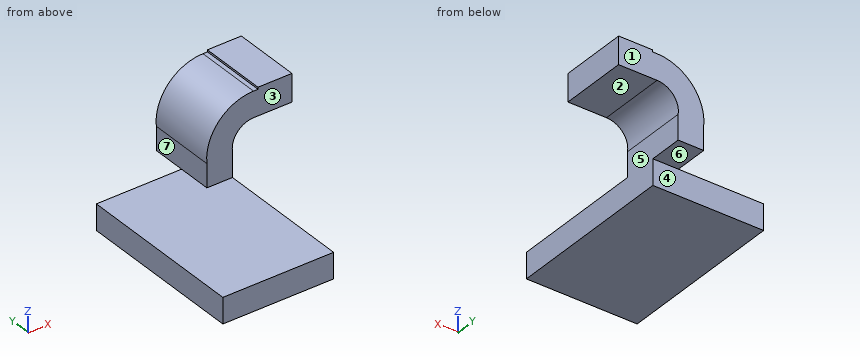
from build123d import *

# Parameters (mm, degrees)
F1_DEPTH = 127
F2_DEPTH = 25.4


with BuildPart() as f1:
    # F0 (on Front) → F1 (new body)
    with BuildSketch(Plane.XZ):
        Polygon((41.275, -9.525), (41.275, 9.525), (22.225, 9.525), (-41.275, 9.525), (-41.275, -9.525), align=None)
    extrude(amount=F1_DEPTH)

    # F0 (on Front) → F2 (join, symmetric)
    with BuildSketch(Plane.XZ):
        with BuildLine():
            Line((22.225, 9.525), (41.275, 9.525))
            Line((41.275, 9.525), (41.275, 27.979645))
            ThreePointArc((41.275, 27.979645), (44.97222, 40.659064), (56.982722, 46.153145))
            Line((56.982722, 46.153145), (60.325, 46.153145))
            Line((60.325, 46.153145), (60.325, 65.203145))
            Line((60.325, 65.203145), (56.982722, 65.203145))
            ThreePointArc((56.982722, 65.203145), (31.108074, 53.735729), (22.225, 26.863997))
            Line((22.225, 26.863997), (22.225, 9.525))
        make_face()
        Polygon((60.325, 65.203145), (60.325, 46.153145), (85.689964, 46.153145), (85.600682, 66.675), (60.325, 66.675), align=None)
    extrude(amount=F2_DEPTH, both=True)


solid = f1.part
The model under review builds one solid part; all positions refer to its coordinate system, in mm. Face numbers are marked on the shaded views. A direction names the side the tool comes from. Round coordinates to 2 decimals unless told otherwise and drop trailing zeros. Loops run counter-clockwise (first coordinate to the right, second up) from the corner with the lowest first, then second, coordinate; pieces in that order, holes last. Notation, with made-up numbers: (80.25, 15.5) -> (84.25, 15.5) arc R16 cw to (84.25, 32.5) -> close; hole circle Ø5 at (14, -11). An arc over 180 degrees is marked (long way). One line per question, with ' | ' between items. Start each with the question number.
Item 1: Add section C-C, the plane z = 18. Write out the cut boundary in (x, y) (3 decimals).
Item 2: Draft analysis for pull direction Z (two halves, no side actions). For the marked faces 5, 6 and 7, state which applies: +Z half, -Z half, draft (parallel to the pull), parting line (faces both ways), or undercut.
Item 3: Machinability: for the marked faces 1, 2, 3 and 4, which of the approach directions +Z, -Z, +X, -X, +Y, -Y give a long, thin tool a straight path to every point of the face, cutting with its end or side? Answer none if there is none.
Item 4: Wall thickness on line 1 along Z through (x, y) = (37.5, -52) (3 decimals); line 2 along X through (y, z) = (-118, 9) (3 decimals); line 3 along Y through (x, z) = (23.5, -5.5): over which ranges is each line inside the solid? List them lowest first. Write a range as [from, to].
Item 5: Add section B-B, the plane x = -27.5. Write out the cut boundary in (y, z) (3 decimals), then the cut area to 3 significant figures.
Item 6: For pin 1 (12 mm diameter, centred on x = 26.5, z = 51.5, fed in from +Y); pin 2 (21 mm diameter, centred on x = -7.5, z = -3.5, fed in from +Y); pin 3 (5 mm diameter, centred on y = 4, z = 18.5, fed in from -X) (3 decimals); pin 4 (9.5 mm diameter, centred on x = 32.5, y = 8.5, fed in from -Z) (3 decimals), all flat-tipped, find the tip position at first contact; note any pin that passes through.
Item 7: Add section A-A, the plane y = -5. Write out the cut boundary in (x, z) (3 decimals).
Return value:
1) outline: (22.225, -25.4) -> (41.275, -25.4) -> (41.275, 25.4) -> (22.225, 25.4) -> close
2) face 5: draft | face 6: -Z half | face 7: undercut
3) face 1: +Z, -Z, +X, -X, +Y | face 2: -Z, +X, +Y, -Y | face 3: +Z, +X, -X, -Y | face 4: -Z, +X, -X, +Y
4) line 1: z = [-9.525, 9.525] | line 2: x = [-41.275, 41.275] | line 3: y = [-127, 0]
5) outline: (-127, -9.525) -> (0, -9.525) -> (0, 9.525) -> (-127, 9.525) -> close | area: 2,420 mm2
6) pin 1: stops at y = 25.4 | pin 2: stops at y = 0 | pin 3: stops at x = 22.225 | pin 4: stops at z = 9.525
7) outline: (-41.275, -9.525) -> (41.275, -9.525) -> (41.275, 27.98) arc R15.875 cw to (56.983, 46.153) -> (85.69, 46.153) -> (85.601, 66.675) -> (60.325, 66.675) -> (60.325, 65.203) -> (56.983, 65.203) arc R34.925 ccw to (22.225, 26.864) -> (22.225, 9.525) -> (-41.275, 9.525) -> close
